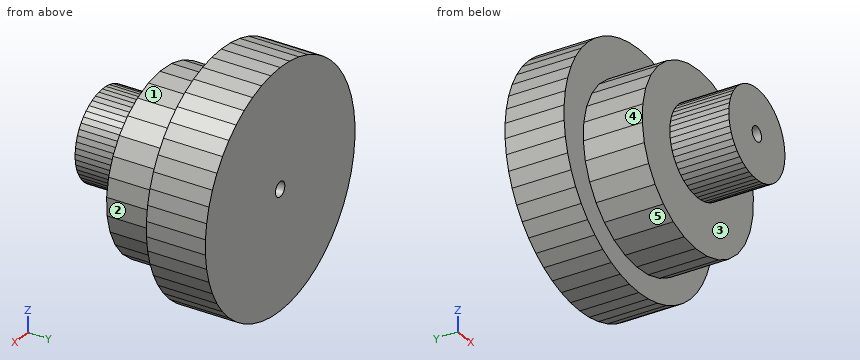
```python
from build123d import *

# Parameters (mm, degrees)
F1_DEPTH = 25.4
F3_DEPTH = 25.4
F5_DEPTH = 25.4
F7_D     = 6.35


with BuildPart() as f1:
    # F0 (on Front) → F1 (new body)
    with BuildSketch(Plane.XZ):
        Polygon((50.8, -3.196065), (50.8, 3.196065), (49.998854, 9.537791), (48.409196, 15.729101), (46.056095, 21.672353), (42.976663, 27.27382), (39.219463, 32.445162), (34.843749, 37.104824), (29.918528, 41.179321), (24.521474, 44.604396), (18.737702, 47.326033), (12.658425, 49.301309), (6.379517, 50.499075), (0, 50.90044), (-6.379517, 50.499075), (-12.658425, 49.301309), (-18.737702, 47.326033), (-24.521474, 44.604396), (-29.918528, 41.179321), (-34.843749, 37.104824), (-39.219463, 32.445162), (-42.976663, 27.27382), (-46.056095, 21.672353), (-48.409196, 15.729101), (-49.998854, 9.537791), (-50.8, 3.196065), (-50.8, -3.196065), (-49.998854, -9.537791), (-48.409196, -15.729101), (-46.056095, -21.672353), (-42.976663, -27.27382), (-39.219463, -32.445162), (-34.843749, -37.104824), (-29.918528, -41.179321), (-24.521474, -44.604396), (-18.737702, -47.326033), (-12.658425, -49.301309), (-6.379517, -50.499075), (0, -50.90044), (6.379517, -50.499075), (12.658425, -49.301309), (18.737702, -47.326033), (24.521474, -44.604396), (29.918528, -41.179321), (34.843749, -37.104824), (39.219463, -32.445162), (42.976663, -27.27382), (46.056095, -21.672353), (48.409196, -15.729101), (49.998854, -9.537791), align=None)
    extrude(amount=F1_DEPTH)

    # F2 (on face) → F3 (join)
    with BuildSketch(Plane.XZ.offset(25.4)):
        Polygon((31.971438, -23.357266), (35.474816, -16.268379), (37.427775, -8.606008), (37.744961, -0.705035), (36.412511, 7.08923), (33.488659, 14.436139), (29.101192, 21.014597), (23.441863, 26.537095), (16.758013, 30.762272), (9.341757, 33.505468), (1.517221, 34.646793), (-6.373624, 34.136364), (-13.985912, 31.996491), (-20.986948, 28.320695), (-27.070754, 23.269627), (-31.971438, 17.064043), (-35.474816, 9.975156), (-37.427775, 2.312784), (-37.744961, -5.588189), (-36.412511, -13.382453), (-33.488659, -20.729362), (-29.101192, -27.30782), (-23.441863, -32.830318), (-16.758013, -37.055495), (-9.341757, -39.798691), (-1.517221, -40.940016), (6.373624, -40.429587), (13.985912, -38.289714), (20.986948, -34.613918), (27.070754, -29.56285), align=None)
    extrude(amount=F3_DEPTH)

    # F4 (on face) → F5 (join)
    with BuildSketch(Plane.XZ.offset(50.8)):
        Polygon((15.820324, -10.638391), (17.02892, -8.571692), (17.96896, -6.369812), (18.625619, -4.067476), (18.98854, -1.700994), (19.052001, 0.692314), (18.815, 3.074704), (18.281276, 5.408604), (17.459245, 7.657207), (16.361871, 9.785051), (15.006461, 11.758579), (13.414389, 13.546667), (11.610765, 15.121116), (9.624033, 16.457097), (7.485523, 17.533539), (5.228962, 18.333466), (2.889938, 18.844264), (0.505337, 19.057877), (-1.887233, 18.970935), (-4.25004, 18.584811), (-6.545822, 17.905593), (-8.738372, 16.943993), (-10.793113, 15.715176), (-12.677639, 14.238521), (-14.362232, 12.537317), (-15.820324, 10.638391), (-17.02892, 8.571692), (-17.96896, 6.369812), (-18.625619, 4.067476), (-18.98854, 1.700994), (-19.052001, -0.692314), (-18.815, -3.074704), (-18.281276, -5.408604), (-17.459245, -7.657207), (-16.361871, -9.785051), (-15.006461, -11.758579), (-13.414389, -13.546667), (-11.610765, -15.121116), (-9.624033, -16.457097), (-7.485523, -17.533539), (-5.228962, -18.333466), (-2.889938, -18.844264), (-0.505337, -19.057877), (1.887233, -18.970935), (4.25004, -18.584811), (6.545822, -17.905593), (8.738372, -16.943993), (10.793113, -15.715176), (12.677639, -14.238521), (14.362232, -12.537317), align=None)
    extrude(amount=F5_DEPTH)

    # F7 (through all)
    with Locations(Plane.XZ.offset(76.2)):
        with Locations((0, 0)):
            Hole(F7_D / 2)


solid = f1.part
```
Source: CAD feature listing. Evaluate the final solid. Frame: model axes, mm. Face numbers are marked on the shaded views. A direction names the side the tool comes from. Give positions to 0.01 mm unless a question says otherwise; leave off trailing zeros. Put each result on its own line as item: value.
Q1. Line query: probe 1 along Z at (x, y) = (0, -20) (3 decimals); probe 2 along Y at (x, z) = (-24.5, 0); probe 3 along Y at (x, z) = (-31, -38). Output: solid intervals per line, ascending. Write a range as [from, to].
Response values:
probe 1: z = [-50.9, -3.175], [3.175, 50.9]
probe 2: y = [-50.8, 0]
probe 3: y = [-25.4, 0]
Q2. Reachability of the marked faces 1, 2, 3, 4 and 5 from +Z, -Z, +X, -X, +Y, -Y: full face, straight path, thin tool, end or side. Return the list, or none.
Response values:
face 1: +Z, +X, -Y
face 2: -Z, +X, -Y
face 3: -Y
face 4: +Z, -X, -Y
face 5: -Z, -X, -Y
Q3. Pin query (flat end, axial travel): P1, Ø10, axis at x = 25.5, y = -58.5, coming from the +Z side; P2, Ø3, axis at x = 24, z = -33, coming from the -Y side; P3, Ø8, axis at y = -43.5, z = -15.5, coming from the +X side; P4, Ø5, axis at x = -5, y = -23, coming from the -Z side. Return the tip coordinate at first contact, or that it passes through.
Response values:
P1: passes through
P2: stops at y = -50.8
P3: stops at x = 36.69
P4: stops at z = -50.74
